CAD build for the part. Positions are in the model's coordinates, mm. Give positions to 0.01 mm unless a question says otherwise; leave off trailing zeros. Loops run counter-clockwise (first coordinate to the right, second up) from the corner with the lowest first, then second, coordinate; pieces in that order, holes last. Notation, with made-up numbers: M -18.75,9 L -7.75,9 A20 cw -7.75,32 Z; hole C -22,45.5 d9. An arc over 180 degrees is marked long. Answer as CSV lines item,"result".
from build123d import *

# Parameters (mm, degrees)
CROQUIS1_R              = 12
CROQUIS1_R_2            = 4
SALIENTE_EXTRUIR1_DEPTH = 8
REDONDEO1_R             = 0.5


with BuildPart() as part:
    # Croquis1 → Saliente-Extruir1 (new body)
    with BuildSketch(Plane.XY):
        Circle(CROQUIS1_R)
        Circle(CROQUIS1_R_2, mode=Mode.SUBTRACT)
    extrude(amount=SALIENTE_EXTRUIR1_DEPTH)

    # Redondeo1
    redondeo1_edges = [part.edges().sort_by_distance(p)[0] for p in [
        (-12, 0, 0),
        (-12, 0, 8),
        (-4, 0, 0),
        (-4, 0, 8),
    ]]
    fillet(redondeo1_edges, radius=REDONDEO1_R)


solid = part.part
1) Band-saw the part on A-A on y = 0. Give the cut face in (x, z).
Answer below:
outline,"M -12,0.5 A0.5 ccw -11.5,0 L -4.5,0 A0.5 ccw -4,0.5 L -4,7.5 A0.5 ccw -4.5,8 L -11.5,8 A0.5 ccw -12,7.5 Z; M 4,0.5 A0.5 ccw 4.5,0 L 11.5,0 A0.5 ccw 12,0.5 L 12,7.5 A0.5 ccw 11.5,8 L 4.5,8 A0.5 ccw 4,7.5 Z"
2) Flat gauge pins, fed straight in: pin 1 (1 mm diameter, centred on x = -7, z = 1.5, fed in from -Y); pin 2 (4 mm diameter, centred on y = 5, z = 1, fed in from +X); pin 3 (3 mm diameter, centred on x = -3, z = 1, fed in from +Y); pin 4 (4 mm diameter, centred on x = 8.5, y = 8.5, fed in from +Z). Where does each tip first touch, or does it go through?
Answer below:
pin 1,"stops at y = -10.09"
pin 2,"stops at x = 11.62"
pin 3,"stops at y = 11.91"
pin 4,"stops at z = 8"
3) Band-saw the part on C-C on z = 2.75. Give the cut face in (x, y), and give its area (3 significant figures).
Answer below:
outline,"C 0,0 d24; hole C 0,0 d8"
area,"402 mm^2"
4) Drill centre lines: line 1 (Y direction, x = 0, z = 2); line 2 (X direction, y = 0.25, z = 3.75); line 3 (X direction, y = 3, z = 5.75). Where is each one in solid material? Low to high. Write a range as from..to.
Answer below:
line 1,"y = -12..-4, 4..12"
line 2,"x = -12..-3.99, 3.99..12"
line 3,"x = -11.62..-2.65, 2.65..11.62"
5) Mould opens along X. For faces 1 (the face through (-0.867, -3.905, 3.951)), 2 (the face through (5, 0, 8)), 3 (the face through (-11.99, 0.53, 3.95)) say: +X half, -X half, draft (parallel to the pull), parting line (faces both ways), or undercut.
Answer below:
face 1,"undercut"
face 2,"draft"
face 3,"parting line"
